Part model, mm, in its own coordinate system. A direction names the side the tool comes from. Give positions to 0.01 mm unless a question says otherwise; leave off trailing zeros. Write each loop counter-clockwise with the first axis right and the second up, starting at its lowest first coordinate (ties: lowest second). Pieces come first, ordered by that corner, then holes. Notation, with made-up numbers: M 82.25,-16 L 121.25,-16 A30 cw 121.25,12 Z; hole C 76,39 d11. An arc over 180 degrees is marked long. Use a Markdown table: item, result. Add a question column.
from build123d import *

# Parameters (mm, degrees)
SKETCH005_R     = 5
PAD002_DEPTH    = 14
SKETCH006_R     = 6
PAD003_DEPTH    = 0.35
SKETCH007_R     = 8
PAD004_DEPTH    = 2
SKETCH008_R     = 0.5
POCKET003_DEPTH = 2


with BuildPart() as part:
    # Sketch005 → Pad002 (new body, symmetric)
    with BuildSketch(Plane.YZ):
        Circle(SKETCH005_R)
    extrude(amount=PAD002_DEPTH, both=True)

    # Sketch006 (on DatumPlane) → Pad003 (new body)
    with BuildSketch(Plane.YZ.offset(13.65)):
        Circle(SKETCH006_R)
    pad003 = extrude(amount=PAD003_DEPTH)

    # Mirrored: Pad003 across YZ
    add(pad003.mirror(Plane.YZ))

    # Sketch007 (on DatumPlane) → Pad004 (new body)
    with BuildSketch(Plane.YZ.offset(13.65)):
        Circle(SKETCH007_R)
    pad004 = extrude(amount=-PAD004_DEPTH)

    # Mirrored001: Pad004 across YZ
    add(pad004.mirror(Plane.YZ))

    # Sketch008 (on DatumPlane) → Pocket003 (cut)
    with BuildSketch(Plane.YZ.offset(13.65)):
        with Locations((-4.949747, 4.949747)):
            Circle(SKETCH008_R)
        with Locations((4.949747, 4.949747)):
            Circle(SKETCH008_R)
        with Locations((4.949747, -4.949747)):
            Circle(SKETCH008_R)
        with Locations((-4.949747, -4.949747)):
            Circle(SKETCH008_R)
    pocket003 = extrude(amount=-POCKET003_DEPTH, mode=Mode.SUBTRACT)

    # Mirrored002: Pocket003 across YZ
    add(pocket003.mirror(Plane.YZ), mode=Mode.SUBTRACT)


solid = part.part
1. Flat gauge pins, fed straight in: pin 1 (8 mm diameter, centred on x = 2.5, y = -5.5, fed in from +Z); pin 2 (5 mm diameter, centred on x = -8, y = 0, fed in from +Z); pin 3 (3 mm diameter, centred on x = -6, z = -1, fed in from +Y); pin 4 (2 mm diameter, centred on y = -3, z = 5.5, fed in from -X). Where does each tip first touch, or does it go through?
2. Cut at B-B (z = -7). Write the cut outline in (x, y), then the cut area to 3 significant figures.
3. Cut at C-C (y = 0). Write the cut outline in (x, z), then the cut area to 3 significant figures.
4. Cut at D-D (x = 3.75). Write the cut outline in (y, z).
5. Mould opens along Y. For faces 5 (the cylindrical face through (13.823, -5.994, 0.264)), 6 (the cylindrical face through (12.664, -5.015, 5.445)), 7 (the cylindrical face through (12.664, -5.015, -4.454)), 8 (the flat face through (-11.65, 5.2, 0.1)) say: released by +Y, released by -Y, zero draft, split by the parting line, or undercut.
6. Drill centre lines: probe 1 along X at (y, z) = (-7.25, -0.75); probe 2 along X at (y, z) = (-5.75, 1.25); probe 3 along Z at (x, y) = (8.25, 0.25). Where is each one in solid material? Low to high. Write a range as [from, to].
7. Cut at A-A (y = 6.5). Write the cut outline in (x, z).
8. Tool access for faces 1 (the cylindrical face through (12.664, 4.581, 5.288)), 2 (the flat face through (11.65, 5.2, 0.1)), 3 (the flat face through (13.65, 2, -6)), 4 (the cylindrical face through (-13.823, -5.994, 0.264)): list every direction of +Z, -Z, +X, -X, +Y, -Y with a clear straight run to the whole face (end or side of a thin tool).
A:
| question | item | result |
|---|---|---|
| 1 | pin 1 | stops at z = 4.77 |
| 1 | pin 2 | stops at z = 5 |
| 1 | pin 3 | stops at y = 5 |
| 1 | pin 4 | stops at x = -14 |
| 2 | outline | M -13.65,-3.87 L -11.65,-3.87 L -11.65,3.87 L -13.65,3.87 Z; M 11.65,-3.87 L 13.65,-3.87 L 13.65,3.87 L 11.65,3.87 Z |
| 2 | area | 31.0 mm² |
| 3 | outline | M -14,-6 L -13.65,-6 L -13.65,-8 L -11.65,-8 L -11.65,-5 L 11.65,-5 L 11.65,-8 L 13.65,-8 L 13.65,-6 L 14,-6 L 14,6 L 13.65,6 L 13.65,8 L 11.65,8 L 11.65,5 L -11.65,5 L -11.65,8 L -13.65,8 L -13.65,6 L -14,6 Z |
| 3 | area | 305 mm² |
| 4 | outline | C 0,0 d10 |
| 5 | face 5 | split by the parting line |
| 5 | face 6 | undercut |
| 5 | face 7 | undercut |
| 5 | face 8 | zero draft |
| 6 | probe 1 | x = [-13.65, -11.65], [11.65, 13.65] |
| 6 | probe 2 | x = [-14, -11.65], [11.65, 14] |
| 6 | probe 3 | z = [-4.99, 4.99] |
| 7 | outline | M -13.65,-4.66 L -11.65,-4.66 L -11.65,4.66 L -13.65,4.66 Z; M 11.65,-4.66 L 13.65,-4.66 L 13.65,4.66 L 11.65,4.66 Z |
| 8 | face 1 | +X, -X |
| 8 | face 2 | none |
| 8 | face 3 | +X |
| 8 | face 4 | -X |
